Design review of the part built by this model. Coordinates are the model's own, in mm. Face numbers are marked on the shaded views. A direction names the side the tool comes from. Coordinates: 2 decimals unless noted, no trailing zeros. Loops run counter-clockwise (first coordinate to the right, second up) from the corner with the lowest first, then second, coordinate; pieces in that order, holes last.
Q1. Add section C-C on y = -1.5. Give the boundary of the cut face in (x, z), and give its area (3 significant figures).
Q2. Add section A-A on y = -6.5. Give the boundary of the cut face in (x, z).
Q3. Wall thickness on probe 1 along Z at (x, y) = (69, -16.5); probe 2 along X at (y, z) = (-23, -6.75): over which ranges is each line inside the solid? List them lowest first.
Q4. For P1, Ø2.5, axis at x = 70, y = -8.5, coming from the -Z side; P2, Ø2.5, axis at x = 70, y = -14.5, coming from the +Z side, all flat-tipped, find the tip position at first contact; note any pin that passes through.
Q5. Machinability: for the marked faces 1 and 2, which of the approach directions +Z, -Z, +X, -X, +Y, -Y give a long, thin tool a straight path to every point of the face, cutting with its end or side? Answer none if there is none.
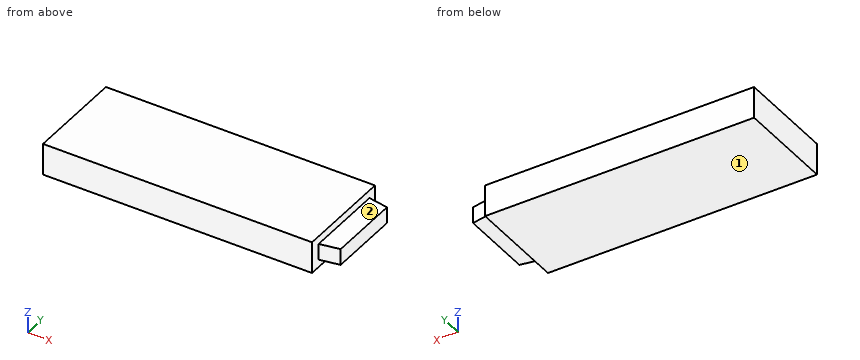
```python
from build123d import *

# Parameters (mm, degrees)
SKETCH1_W           = 68
SKETCH1_H           = 25
BOSS_EXTRUDE1_DEPTH = 8
SKETCH13_W          = 4.102736362
SKETCH13_H          = 20.181027508
BOSS_EXTRUDE5_DEPTH = 5
CHAMFER1_SIZE2      = 0.881634904
CHAMFER1_SIZE       = 5
CHAMFER2_SIZE2      = 5
CHAMFER2_SIZE       = 0.881634904


with BuildPart() as part:
    # Sketch1 → Boss-Extrude1 (new body)
    with BuildSketch(Plane(origin=(0, 0, 0), x_dir=(1, 0, 0), z_dir=(0, 0, -1))):
        with Locations((34, 12.5)):
            Rectangle(SKETCH1_W, SKETCH1_H)
    extrude(amount=BOSS_EXTRUDE1_DEPTH)

    # Sketch13 → Boss-Extrude5 (add)
    with BuildSketch(Plane(origin=(68, 0, 0), x_dir=(0, 0, -1), z_dir=(1, 0, 0))):
        with Locations((4.036961589, -12.278230467)):
            Rectangle(SKETCH13_W, SKETCH13_H)
    extrude(amount=BOSS_EXTRUDE5_DEPTH)

    # Chamfer1
    chamfer1_edges = [part.edges().sort_by_distance(p)[0] for p in [
        (73, -2.187716713, -4.036961589),
    ]]
    chamfer1_side = [part.faces().sort_by_distance(p)[0] for p in [
        (72.982367302, -2.187716713, -4.036961589),
    ]]
    chamfer(chamfer1_edges, length=CHAMFER1_SIZE - 0.0001, length2=CHAMFER1_SIZE2 - 0.0001, reference=chamfer1_side[0])  # a hair under: the kernel refuses the full size

    # Chamfer2
    chamfer2_edges = [part.edges().sort_by_distance(p)[0] for p in [
        (73, -22.368744221, -4.036961589),
    ]]
    chamfer2_side = [part.faces().sort_by_distance(p)[0] for p in [
        (73, -22.351111523, -4.036961589),
    ]]
    chamfer(chamfer2_edges, length=CHAMFER2_SIZE - 0.0001, length2=CHAMFER2_SIZE2 - 0.0001, reference=chamfer2_side[0])  # a hair under: the kernel refuses the full size


solid = part.part
```
Entries:
1. outline: (0, -8) - (68, -8) - (68, 0) - (0, 0) - close
1. area: 544 mm2
2. outline: (0, -8) - (68, -8) - (68, -6.09) - (73, -6.09) - (73, -1.99) - (68, -1.99) - (68, 0) - (0, 0) - close
3. probe 1: z = -6.09 to -1.99
3. probe 2: x = 0 to 68
4. P1: stops at z = -6.09
4. P2: stops at z = -1.99
5. face 1: -Z, +X, -X, +Y, -Y
5. face 2: +Z, +X, +Y, -Y
